```python
from build123d import *

# Parameters (mm, degrees)
SKETCH_1_W      = 400
SKETCH_1_H      = 200
SKETCH_1_W_2    = 200
SKETCH_1_H_2    = 400
EXTRUDE_1_DEPTH = 200


with BuildPart() as part:
    # 草圖1 → 填料-伸長1 (new body)
    with BuildSketch(Plane(origin=(0, 0, 0), x_dir=(1, 0, 0), z_dir=(0, 1, 0))):
        with Locations((-300, 0)):
            Rectangle(SKETCH_1_W, SKETCH_1_H)
        Rectangle(SKETCH_1_W_2, SKETCH_1_H)
        with Locations((300, 0)):
            Rectangle(SKETCH_1_W, SKETCH_1_H)
        with Locations((0, -300)):
            Rectangle(SKETCH_1_W_2, SKETCH_1_H_2)
        with Locations((0, 300)):
            Rectangle(SKETCH_1_W_2, SKETCH_1_H_2)
    extrude(amount=EXTRUDE_1_DEPTH)


solid = part.part
```
Work out the finished part from the listing and answer in its coordinate system (mm). A direction names the side the tool comes from. Round coordinates to 2 decimals unless told otherwise and drop trailing zeros. Write each loop counter-clockwise with the first axis right and the second up, starting at its lowest first coordinate (ties: lowest second). Pieces come first, ordered by that corner, then holes. Notation, with made-up numbers: (60, 0) -> (114, 0) arc R12 ccw to (114, 5) -> close; hole circle Ø3 at (67, -9). An arc over 180 degrees is marked (long way). Write each question's results on one line, items separated by ' | '.
Q1. Section C-C, the plane z = 404 is taken. Write down the section's boundary in (x, y).
Data:
outline: (-100, 0) -> (100, 0) -> (100, 200) -> (-100, 200) -> close
Q2. Determine the mould class of faces 5 (the flat face through (-1, 99, 500)), 6 (the flat face through (-39, 200, -2)), 7 (the flat face through (-297, 99, -100)) for opening direction Z: released by +Z, released by -Z, zero draft, split by the parting line, or undercut.
Data:
face 5: released by +Z | face 6: zero draft | face 7: released by -Z
Q3. A straight line is drawn through the part: line 1 along X through (y, z) = (72, -323). Find the intervals that lie inside material, in ascending order. Write a range as [from, to].
Data:
line 1: [-100, 100]
Q4. Section B-B, the plane x = 323.5 is taken. Write down the section's boundary in (y, z).
Data:
outline: (0, -100) -> (200, -100) -> (200, 100) -> (0, 100) -> close
Q5. Section A-A, the plane y = 112 is taken. Write down the section's boundary in (x, z).
Data:
outline: (-500, -100) -> (-100, -100) -> (-100, -500) -> (100, -500) -> (100, -100) -> (500, -100) -> (500, 100) -> (100, 100) -> (100, 500) -> (-100, 500) -> (-100, 100) -> (-500, 100) -> close
Q6. A flat-ended cylindrical pin translates along its axis: P1, Ø10, axis at y = 48, z = -194, coming from the -X side. Find the tip coordinate at first contact, or state that the pin passes through.
Data:
P1: x = -100
Q7. Which of the six approach directions +Z, -Z, +X, -X, +Y, -Y give full straight-line access (tool end or side, diameter ignored) to faces 1 (the flat face through (100, 99, 303)), 2 (the flat face through (-303, 99, 100)), 3 (the flat face through (100, 99, -297)), 4 (the flat face through (-100, 99, -297))?
Data:
face 1: +Z, +X, +Y, -Y | face 2: +Z, -X, +Y, -Y | face 3: -Z, +X, +Y, -Y | face 4: -Z, -X, +Y, -Y
